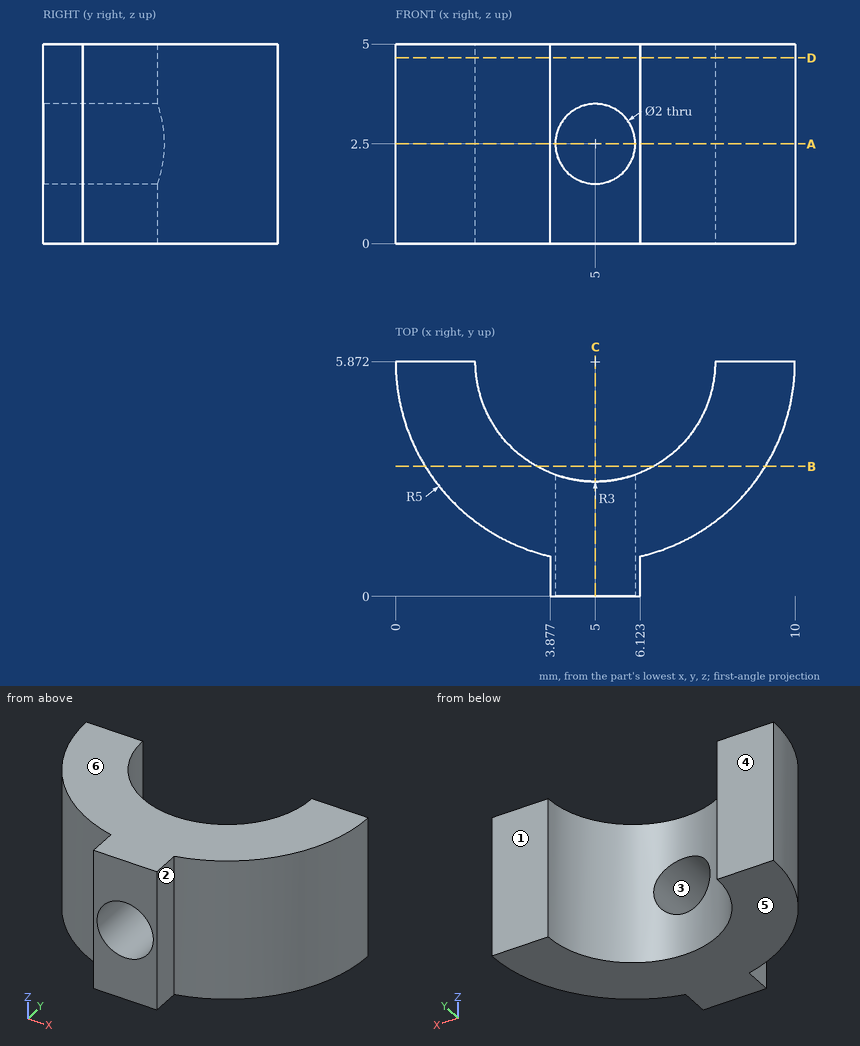
For this review, use the dimensioned drawing (mm, ordinates from the lowest corner) and the shaded views. A direction names the side the tool comes from. Give positions to 0.01 mm unless a question says otherwise; leave off trailing zeros. Order: outer loops, then holes, each group sorted by start corner. A loop starts at its lowest first (then second) coordinate and runs counter-clockwise, first axis right, second up. Notation, with made-up numbers: M -1.75,37.5 L 19.25,37.5 A21 cw 19.25,68.5 Z; hole C 50,25 d1. An arc over 180 degrees is marked long. One line per question, with ' | ' between items. Start each with the question number.
1) Consider section D-D, the plane z = 4.65. Give the boundary of the cut face in (x, y).
2) Clearance check with flat-ended pins moving along their axes: P1, Ø1, axis at y = 2, z = 0.5, coming from the +X side; P2, Ø1, axis at y = 3, z = 4.5, coming from the -X side; P3, Ø3, axis at x = 1.5, z = 4.5, coming from the -Y side. State where each tip first meets the part, or that it passes through.
3) Consider section C-C, the plane x = 5. Give the boundary of the cut face in (y, z).
4) Mouldability with a two-part tool opening along Z and no side actions: class the marked faces 3, 4, 5 and 6 as pulls with the +Z half, pulls with the -Z half, needs draft (parallel to the pull), parting line crosses it, or undercut.
5) For the marked faces 1 and 2, list the 3-axis set-ups (+Z, -Z, +X, -X, +Y, -Y) from which the entire face can be reached by the end or side of a thin tool; tool diameter is ignored.
6) Consider section B-B, the plane y = 3.25. Give the boundary of the cut face in (x, z).
7) Wall thickness on L1, parallel to Z at x = 5, y = 1.5; L2, parallel to Y at x = 1, z = 1.85; L3, parallel to X at y = 3.6, z = 2.4 (1 decimal): over which ranges is each line inside the solid? List them lowest first. Write a range as from..to.
8) Consider section A-A, the plane z = 2.5. Give the boundary of the cut face in (x, y).
Found:
1) outline: M 0,5.87 A5 ccw 3.88,1 L 3.88,0 L 6.12,0 L 6.12,1 A5 ccw 10,5.87 L 8,5.87 A3 cw 2,5.87 Z
2) P1: stops at x = 8.69 | P2: stops at x = 0.6 | P3: stops at y = 1.29
3) outline: M 0,0 L 2.87,0 L 2.87,1.5 L 0,1.5 Z; M 0,3.5 L 2.87,3.5 L 2.87,5 L 0,5 Z
4) face 3: undercut | face 4: needs draft | face 5: pulls with the -Z half | face 6: pulls with the +Z half
5) face 1: +Z, -Z, +X, -X, +Y | face 2: +Z, -Z, +X, -Y
6) outline: M 0.74,0 L 3.54,0 L 3.54,5 L 0.74,5 Z; M 6.46,0 L 9.26,0 L 9.26,5 L 6.46,5 Z
7) L1: z = 0..1.5, 3.5..5 | L2: y = 2.87..5.87 | L3: x = 0.5..3, 7..9.5
8) outline: M 0,5.87 A5 ccw 3.88,1 L 3.88,0 L 4,0 L 4,3.04 A3 cw 2,5.87 Z; M 6,0 L 6.12,0 L 6.12,1 A5 ccw 10,5.87 L 8,5.87 A3 cw 6,3.04 Z
